For this review, take the finished solid that the model builds, in its own axes (mm). Face numbers are marked on the shaded views. Coordinates: 2 decimals unless noted, no trailing zeros. Order: outer loops, then holes, each group sorted by start corner. A loop starts at its lowest first (then second) coordinate and runs counter-clockwise, first axis right, second up. Notation, with made-up numbers: (10, 23) -> (27, 23) arc R18 cw to (27, 56) -> close; hole circle Ø4 at (13, -27.5). An arc over 180 degrees is marked (long way). Return JSON: item names as keys, results as strings. Group by question number.
Item 1: Take a section at B-B (z = 16). Write out the cut boundary in (x, y).
Item 2: Insertion check: pin 1 (12 mm diameter, centred on x = -2, z = 23, fed in from +Y). The pin has a flat end and moves straight along its axis. Give the tip position at first contact, or say it passes through.
Item 3: Take a section at D-D (z = 22.5). Write out the cut boundary in (x, y).
Item 4: Take a section at C-C (y = 1.95). Write out the cut boundary in (x, z) (3 decimals).
Item 5: For line 1 along Z through (x, y) = (0.5, 1.8); line 2 along Y through (x, z) = (2.5, 28.5); line 3 along X through (y, z) = (2.8, 15), list the stretches that pass through material, from the lowest coordinate up.
Item 6: Draft analysis for pull direction X (two halves, no side actions). For the marked faces 1, 2, 3 and 4, state which applies: +X half, -X half, draft (parallel to the pull), parting line (faces both ways), or undercut.
Item 7: Take a section at A-A (x = 0). Write out the cut boundary in (y, z) (3 decimals), then the cut area to 4 significant figures.
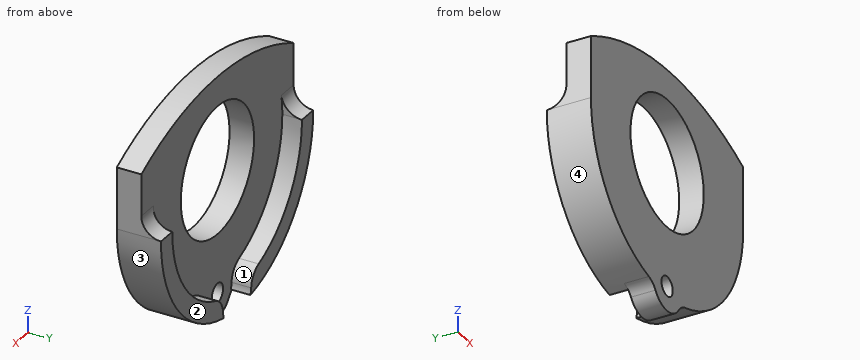
```python
from build123d import *

# Parameters (mm, degrees)
SKETCH1_R                  = 6.5
SKETCH1_R_2                = 1
MAIN_EXTRUDE_DEPTH         = 2.5
BATTERY_START              = 2
BATTERY_RING_CRADDLE_DEPTH = 2
FILLETS_R                  = 2


with BuildPart() as part:
    # Sketch1 → Main extrude (new body)
    with BuildSketch(Plane.XZ.offset(-2.5)):
        with BuildLine():
            Line((-13.5, 26.437647872), (-13.5, 20.185))
            ThreePointArc((-13.5, 20.185), (-10.350618886, 11.518126938), (-2.371897974, 6.895))
            ThreePointArc((-2.371897974, 6.895), (0, 5.185), (2.371897974, 6.895))
            ThreePointArc((2.371897974, 6.895), (10.350618886, 11.518126938), (13.5, 20.185))
            Line((13.5, 20.185), (13.5, 26.437647872))
            ThreePointArc((13.5, 26.437647872), (0, 29.685), (-13.5, 26.437647872))
        make_face()
        with Locations(Location((0, 20.185, 0), (0, 0, 90))):
            Circle(SKETCH1_R, mode=Mode.SUBTRACT)
        with Locations(Location((0, 7.685, 0), (0, 0, 90))):
            Circle(SKETCH1_R_2, mode=Mode.SUBTRACT)
    extrude(amount=MAIN_EXTRUDE_DEPTH)

    # Sketch2 → Battery ring craddle (add)
    with BuildSketch(Plane(origin=(0, 2.5, 0), x_dir=(1, 0, 0), z_dir=(0, 1, 0)).offset(BATTERY_START)):
        with BuildLine():
            Line((-13.5, -20.185), (-11.5, -20.185))
            ThreePointArc((-11.5, -20.185), (-9.38817648, -13.543302748), (-3.828323063, -9.340925926))
            ThreePointArc((-3.828323063, -9.340925926), (-2.89145393, -8.651439161), (-2.496732433, -7.557222222))
            ThreePointArc((-2.496732433, -7.557222222), (-2.456730567, -7.221885627), (-2.371897974, -6.895))
            ThreePointArc((-2.371897974, -6.895), (-10.350618886, -11.518126938), (-13.5, -20.185))
        make_face()
        with BuildLine():
            Line((13.5, -20.185), (11.5, -20.185))
            ThreePointArc((11.5, -20.185), (9.38817648, -13.543302748), (3.828323063, -9.340925926))
            ThreePointArc((3.828323063, -9.340925926), (2.89145393, -8.651439161), (2.496732433, -7.557222222))
            ThreePointArc((2.496732433, -7.557222222), (2.456730567, -7.221885627), (2.371897974, -6.895))
            ThreePointArc((2.371897974, -6.895), (10.350618886, -11.518126938), (13.5, -20.185))
        make_face()
    extrude(amount=-BATTERY_RING_CRADDLE_DEPTH)

    # Fillets
    # the kernel refuses this fillet: 2 mm, written as the material it adds along each edge
    with BuildSketch(Plane(origin=(2.371897974, 2.5, 6.895), x_dir=(-0.4457237071000903, 0, -0.8951705853796543), z_dir=(0, -1, 0))) as fillets_piece_1:
        with BuildLine():
            CenterArc((0.980073907, 1.980300021), FILLETS_R, 220.3095964, 41.641946396)
            ThreePointArc((-0.545046071, 0.686465004), (-0.266950187, 0.347657285), (0, 0))
            ThreePointArc((0, 0), (0.350026395, 0.024624973), (0.700052791, 0))
        make_face()
    extrude(amount=2.5)
    with BuildSketch(Plane(origin=(-2.371897974, 2.5, 6.895), x_dir=(-0.9782217139639082, 0, 0.20756270939047247), z_dir=(0, -1, 0))) as fillets_piece_2:
        with BuildLine():
            CenterArc((0.941460954, 1.9989458), FILLETS_R, 226.497666749, 41.641946396)
            ThreePointArc((-0.435307275, 0.548253123), (-0.198368351, 0.289438878), (0, 0))
            ThreePointArc((0, 0), (0.438266306, 0.007115851), (0.876532612, 0))
        make_face()
    extrude(amount=2.5)
    with BuildSketch(Plane(origin=(-13.5, 2.5, 20.185), x_dir=(0, 0, 1), z_dir=(1, 0, 0))) as fillets_piece_3_section:
        with BuildLine():
            CenterArc((FILLETS_R, -FILLETS_R), FILLETS_R, 90, 90)
            Line((0, -FILLETS_R), (0, 0))
            Line((0, 0), (FILLETS_R, 0))
        make_face()
    fillets_piece_3 = extrude(amount=7, mode=Mode.PRIVATE)
    fillets_piece_3 = fillets_piece_3 - Plane(origin=(0, 2.67362595, 20.185), x_dir=(-1, 0, 0), z_dir=(0, 1, 0)) * Cylinder(11.5, 22, mode=Mode.PRIVATE)
    add(fillets_piece_3)
    with BuildSketch(Plane(origin=(13.5, 2.5, 20.185), x_dir=(0, 0, 1), z_dir=(-1, 0, 0))) as fillets_piece_4_section:
        with BuildLine():
            CenterArc((FILLETS_R, FILLETS_R), FILLETS_R, 180, 90)
            Line((0, FILLETS_R), (0, 0))
            Line((0, 0), (FILLETS_R, 0))
        make_face()
    fillets_piece_4 = extrude(amount=7, mode=Mode.PRIVATE)
    fillets_piece_4 = fillets_piece_4 - Plane(origin=(0, 2.673614475, 20.185), x_dir=(1, 0, 0), z_dir=(0, 1, 0)) * Cylinder(11.5, 22, mode=Mode.PRIVATE)
    add(fillets_piece_4)


solid = part.part
```
Findings below:
{
 "1": {"outline": "(-12.83, 0) -> (-4.97, 0) -> (-4.97, 2.5) -> (-10.71, 2.5) -> (-10.71, 4.5) -> (-12.83, 4.5) -> close; (4.97, 0) -> (12.83, 0) -> (12.83, 4.5) -> (10.71, 4.5) -> (10.71, 2.5) -> (4.97, 2.5) -> close"},
 "2": {"pin 1": "stops at y = 2.5"},
 "3": {"outline": "(-13.5, 0) -> (-6.07, 0) -> (-6.07, 2.5) -> (-13.5, 2.5) -> close; (6.07, 0) -> (13.5, 0) -> (13.5, 2.5) -> (6.07, 2.5) -> close"},
 "4": {"outline": "(-13.5, 20.185) arc R13.5 ccw to (-3.229, 7.077) arc R2 cw to (-2.06, 6.268) arc R2.5 ccw to (2.06, 6.268) arc R2 cw to (3.229, 7.077) arc R13.5 ccw to (13.5, 20.185) -> (13.5, 26.438) arc R29.685 ccw to (-13.5, 26.438) -> close; hole circle Ø13 at (0, 20.185); hole circle Ø2 at (0, 7.685)"},
 "5": {"line 1": "z = 5.24 to 6.82, 8.55 to 13.7, 26.67 to 29.68", "line 2": "y = 0 to 2.5", "line 3": "x = -12.46 to -10.26, 10.26 to 12.46"},
 "6": {"face 1": "undercut", "face 2": "draft", "face 3": "+X half", "face 4": "-X half"},
 "7": {"outline": "(0, 5.185) -> (2.5, 5.185) -> (2.5, 6.685) -> (0, 6.685) -> close; (0, 8.685) -> (2.5, 8.685) -> (2.5, 13.685) -> (0, 13.685) -> close; (0, 26.685) -> (2.5, 26.685) -> (2.5, 29.685) -> (0, 29.685) -> close", "area": "23.75 mm2"}
}
